```python
from build123d import *

# Parameters (mm, degrees)
F1_DEPTH = 40
F2_R     = 5
F3_DEPTH = 65
F4_R     = 2
F5_DEPTH = 40.001


with BuildPart() as f1:
    # F0 (on Front) → F1 (new body)
    with BuildSketch(Plane.XZ):
        Polygon((-84.199729, 0), (-84.199729, -32.299187), (215.800271, -32.299187), (215.800271, -25.689224), (44.751238, 8.807085), (-36.943395, 8.807085), align=None)
    extrude(amount=F1_DEPTH)

    # F2 (on face) → F3 (cut)
    with BuildSketch(Plane(origin=(-84.199729, 0, 0), x_dir=(0, -1, 0), z_dir=(-1, 0, 0))):
        with Locations((20, 2.700813)):
            Circle(F2_R)
    extrude(amount=-F3_DEPTH, mode=Mode.SUBTRACT)

    # F4 (on face) → F5 (cut, through all)
    with BuildSketch(Plane.XZ.offset(40)):
        with Locations((-35.561115, -24.638616)):
            Circle(F4_R)
        with Locations((174.334928, -24.638616)):
            Circle(F4_R)
    extrude(amount=-F5_DEPTH, mode=Mode.SUBTRACT)


solid = f1.part
```
Can you work these out from the model? Positions are in its coordinate system, mm. Give positions to 0.01 mm unless a question says otherwise; leave off trailing zeros. Loops run counter-clockwise (first coordinate to the right, second up) from the corner with the lowest first, then second, coordinate; pieces in that order, holes last. Notation, with made-up numbers: M -19,80 L 18,80 A16 ccw 18,86 Z; hole C 44.5,51.5 d2. An arc over 180 degrees is marked long. One line per question, with ' | ' between items. Start each with the question number.
Q1. For pin 1 Ø8 at (x, y) = (79, -26.5) entering from +Z; pin 2 Ø5 at (y, z) = (-19, 0.5) entering from -X; pin 3 Ø8 at (x, y) = (125, -32.5) entering from +Z; pin 4 Ø12 at (x, z) = (141, -0.5) entering from -Y, each with a flat end and sliding along its axis, tell me the tip position at first contact or that it passes through.
Q2. If we section it at C-C (x = 154.5): Please give me the cut outline in (y, z), plus the area to 3 significant figures.
Q3. If we section it at A-A (y = -20): Please give me the cut outline in (x, z), plus the area to 3 significant figures.
Q4. If we mould it in two halves opening along Z, with no side actions, what happens to faces 1 (the flat face through (30, -40, -16)), 2 (the flat face through (-19.2, -20, 3)), 3 (the cylindrical face through (-44.93, -18.92, -2.18)), 4 (the flat face through (131.47, -19.72, -8.68))? For each: +Z half, -Z half, draft (parallel to the pull), parting line (faces both ways), or undercut.
Q5. If I drill on line 1 (X direction, y = -19.5, z = -26); line 2 (Z direction, x = 85.5, y = -37); line 3 (Z direction, x = 192.5, y = -7.5), over which ranges is the centre line in solid material (lowest first)? Write a range as from..to.
Q6. If we section it at B-B (x = -24): Please give me the cut outline in (y, z), plus the area to 3 significant figures.
Q7. If we section it at D-D (y = -33.5): Please give me the cut outline in (x, z), plus the area to 3 significant figures.
Computed:
1) pin 1: stops at z = 2.71 | pin 2: stops at x = -19.2 | pin 3: stops at z = -6.57 | pin 4: passes through
2) outline: M -40,-32.3 L 0,-32.3 L 0,-13.33 L -40,-13.33 Z | area: 759 mm²
3) outline: M -84.2,-32.3 L 215.8,-32.3 L 215.8,-25.69 L 44.75,8.81 L -36.94,8.81 L -42.88,7.7 L -19.2,7.7 L -19.2,-2.3 L -84.2,-2.3 Z; hole C -35.56,-24.64 d4; hole C 174.33,-24.64 d4 | area: 8,660 mm²
4) face 1: draft | face 2: undercut | face 3: undercut | face 4: +Z half
5) line 1: x = -84.2..-37.03, -34.1..172.87, 175.8..215.8 | line 2: z = -32.3..0.59 | line 3: z = -32.3..-20.99
6) outline: M -40,-32.3 L 0,-32.3 L 0,8.81 L -40,8.81 Z; hole C -20,2.7 d10 | area: 1,570 mm²
7) outline: M -84.2,-32.3 L 215.8,-32.3 L 215.8,-25.69 L 44.75,8.81 L -36.94,8.81 L -84.2,0 Z; hole C -35.56,-24.64 d4; hole C 174.33,-24.64 d4 | area: 9,150 mm²
